Source: three-view drawing plus pictorial views. Frame: mm from the lowest corner of the part. A direction names the side the tool comes from. Coordinates: 2 decimals unless noted, no trailing zeros. Write each loop counter-clockwise with the first axis right and the second up, starting at its lowest first coordinate (ties: lowest second). Pieces come first, ordered by that corner, then holes. Notation, with made-up numbers: M 67,-3 L 71,-3 A23 ccw 71,25 Z; hole C -29,45.25 d4. An arc over 180 degrees is marked long. Write item = value, one per line. Start each with the question number.
Item 1: Section C-C on x = 27. Output: boundary loops of the cut face in (y, z), plus the area to 3 significant figures.
Item 2: Reachability of the marked faces 5, 6 and 7 from +Z, -Z, +X, -X, +Y, -Y: full face, straight path, thin tool, end or side. Return the list, or none.
Item 3: Section A-A on x = 42. Output: boundary loops of the cut face in (y, z).
Item 4: First-contact query: pin 1 Ø2 at (x, y) = (23, 12.5) entering from -Z; pin 2 Ø7.5 at (y, z) = (6.5, 37.5) entering from -X; pin 3 Ø1 at (y, z) = (15.5, 33) entering from +X. Flat tips, straight axial feed; report the tip coordinate or a pass-through.
Item 5: Ray query, L1, parallel to Z at x = 36, y = 9.25; L2, parallel to X at y = 3, z = 10; L3, parallel to Z at x = 18.5, y = 15. Return the intervals inside material, ascending. Write a range as [from, to].
Item 6: Section D-D on z = 43. Output: boundary loops of the cut face in (x, y), plus the area to 3 significant figures.
Item 7: Section B-B on y = 9.25. Output: boundary loops of the cut face in (x, z), plus the area to 3 significant figures.
Item 8: Pull-direction query (Z, two-part tool) for the marked faces 1, 2, 3 and 4; classes: +Z half, -Z half, draft (parallel to the pull), parting line (faces both ways), or undercut.
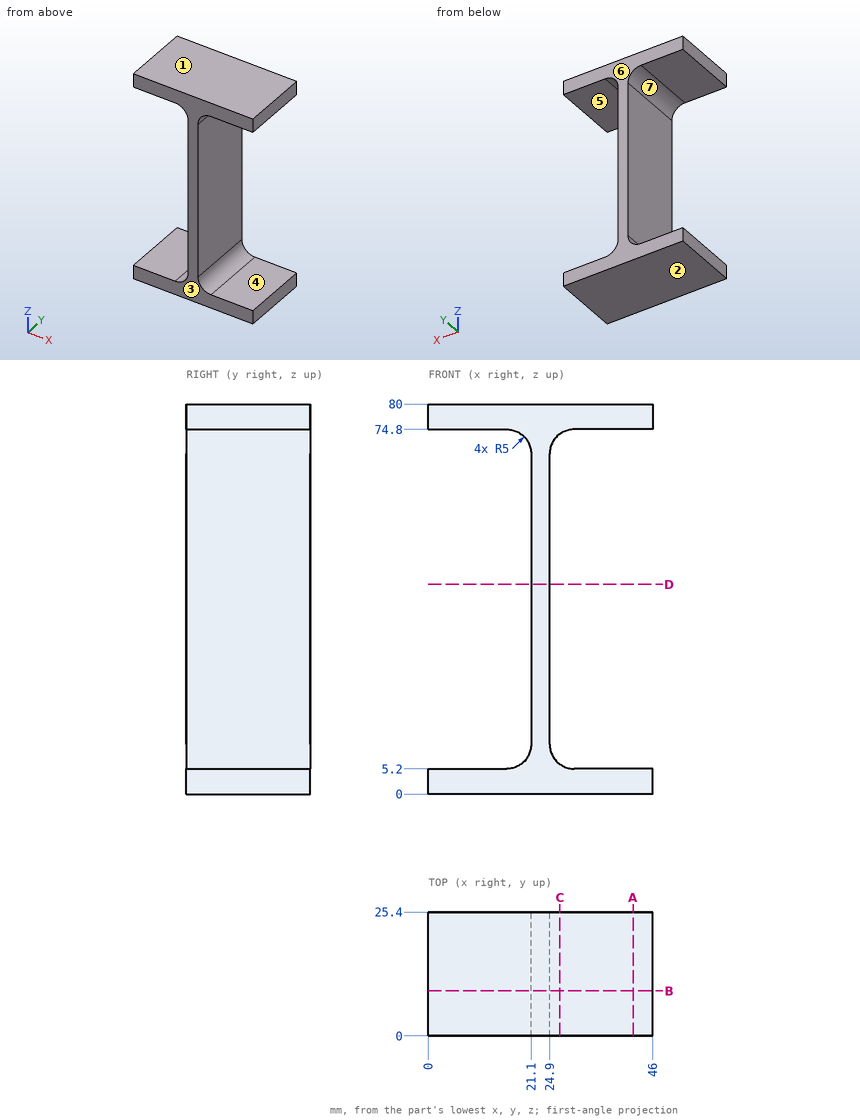
Responses:
q1.outline = M 0,0 L 25.4,0 L 25.4,6.13 L 0,6.13 Z; M 0,73.87 L 25.4,73.87 L 25.4,80 L 0,80 Z
q1.area = 311 mm²
q2.face_5 = +X, +Y, -Y
q2.face_6 = +Z, -Z, +X, -X, +Y
q2.face_7 = -X, +Y, -Y
q3.outline = M 0,0 L 25.4,0 L 25.4,5.2 L 0,5.2 Z; M 0,74.8 L 25.4,74.8 L 25.4,80 L 0,80 Z
q4.pin_1 = 0
q4.pin_2 = 21.1
q4.pin_3 = 24.9
q5.L1 = [0, 5.2], [74.8, 80]
q5.L2 = [21.1, 24.9]
q5.L3 = [0, 5.81], [74.19, 80]
q6.outline = M 21.1,0 L 24.9,0 L 24.9,25.4 L 21.1,25.4 Z
q6.area = 96.5 mm²
q7.outline = M 0,0 L 46,0 L 46,5.2 L 29.9,5.2 A5 cw 24.9,10.2 L 24.9,69.8 A5 cw 29.9,74.8 L 46,74.8 L 46,80 L 0,80 L 0,74.8 L 16.1,74.8 A5 cw 21.1,69.8 L 21.1,10.2 A5 cw 16.1,5.2 L 0,5.2 Z
q7.area = 764 mm²
q8.face_1 = +Z half
q8.face_2 = -Z half
q8.face_3 = draft
q8.face_4 = undercut
